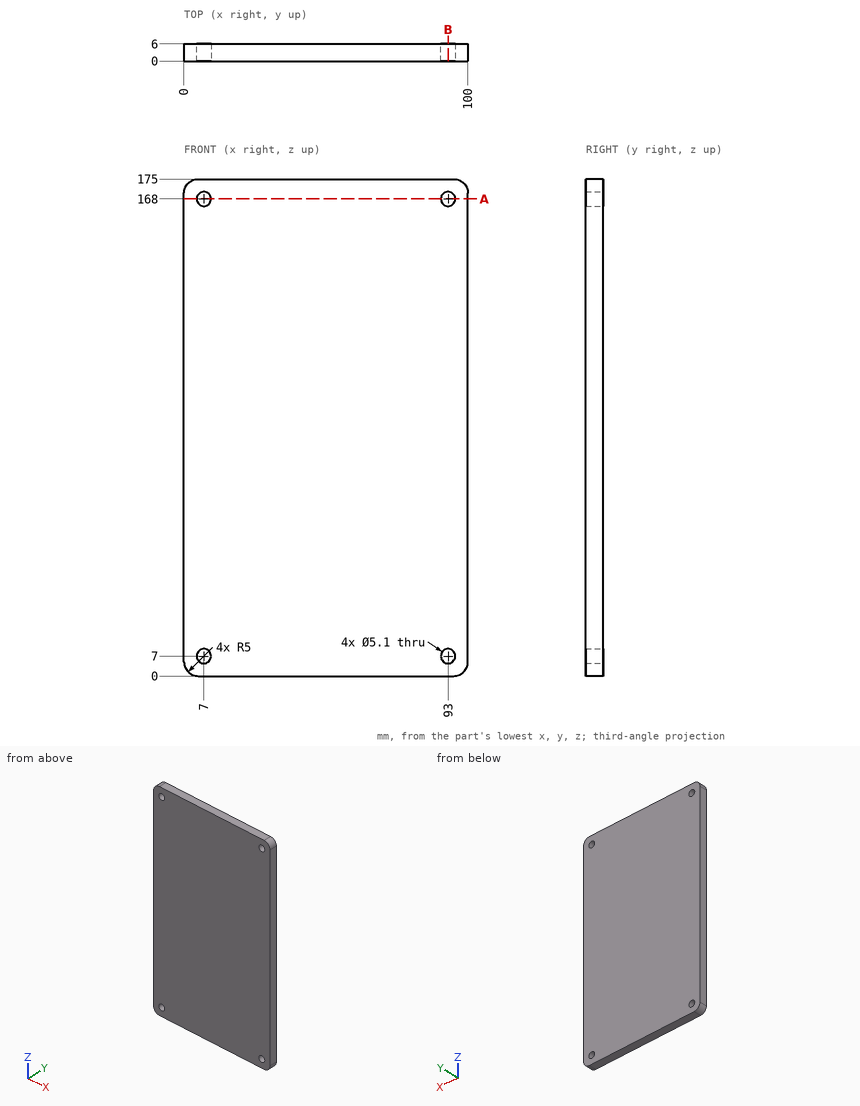
Answer from the drawing. Dimensions are ordinates in mm from the lowest x, y and z of the part. Coordinates: 2 decimals unless noted, no trailing zeros. Loops run counter-clockwise (first coordinate to the right, second up) from the corner with the lowest first, then second, coordinate; pieces in that order, holes last.
1) Section A-A (z = 168) is taken. Give the vertices of the cut face in (x, y), plus the area to 3 significant figures.
Results:
outline: (0, 0) - (4.45, 0) - (4.45, 6) - (0, 6) - close; (9.55, 0) - (90.45, 0) - (90.45, 6) - (9.55, 6) - close; (95.55, 0) - (100, 0) - (100, 6) - (95.55, 6) - close
area: 539 mm2
2) A flat-ended cylindrical pin translates along its axis: pin 1 (6.5 mm diameter, centred on x = 93, z = 168, fed in from +Y). Find the tip coordinate at first contact, or state that the pin passes through.
Results:
pin 1: stops at y = 6
3) Consider probe 1 along Z at (x, y) = (7, 3.1); probe 2 along X at (y, z) = (3.25, 168). Determine where each line is inside the solid, lowest interval first.
Results:
probe 1: z = 0 to 4.45, 9.55 to 165.45, 170.55 to 175
probe 2: x = 0 to 4.45, 9.55 to 90.45, 95.55 to 100
4) Section B-B (x = 93) is taken. Give the vertices of the cut face in (y, z), plus the area to 3 significant figures.
Results:
outline: (0, 0) - (6, 0) - (6, 4.45) - (0, 4.45) - close; (0, 9.55) - (6, 9.55) - (6, 165.45) - (0, 165.45) - close; (0, 170.55) - (6, 170.55) - (6, 175) - (0, 175) - close
area: 989 mm2
